The model under review builds one solid part; all positions refer to its coordinate system, in mm. A direction names the side the tool comes from. Coordinates: 2 decimals unless noted, no trailing zeros. Loops run counter-clockwise (first coordinate to the right, second up) from the corner with the lowest first, then second, coordinate; pieces in that order, holes last. Notation, with made-up numbers: M -29.75,-36.75 L 9.25,-36.75 A12 ccw 9.25,-23.75 Z; hole C 14.25,25.25 d7. An arc over 180 degrees is marked long. Use one line per item in the form item = value.
```python
from build123d import *

# Parameters (mm, degrees)
F0_W      = 33
F0_H      = 10
F1_DEPTH  = 5
F2_R      = 1.75
F3_DEPTH  = 5
F2_R_2    = 3
F4_DEPTH  = 3
F5_W      = 33
F5_H      = 30
F6_DEPTH  = 6
F7_R      = 4
F8_DEPTH  = 6
F9_R      = 1.5
F10_DEPTH = 4.2929008565
F12_DEPTH = 6


with BuildPart() as f1:
    # F0 (on Front) → F1 (new body)
    with BuildSketch(Plane.XZ):
        Rectangle(F0_W, F0_H)
    extrude(amount=F1_DEPTH)

    # F2 (on face) → F3 (cut, through all)
    with BuildSketch(Plane.XZ.offset(5)):
        with Locations((-12, 1)):
            Circle(F2_R)
        with Locations((12, 1)):
            Circle(F2_R)
    extrude(amount=-F3_DEPTH, mode=Mode.SUBTRACT)

    # F2 (on face) → F4 (cut)
    with BuildSketch(Plane.XZ.offset(5)):
        with Locations((-12, 1)):
            Circle(F2_R_2)
        with Locations((-12, 1)):
            Circle(F2_R, mode=Mode.SUBTRACT)
        with Locations((12, 1)):
            Circle(F2_R_2)
        with Locations((12, 1)):
            Circle(F2_R, mode=Mode.SUBTRACT)
    extrude(amount=-F4_DEPTH, mode=Mode.SUBTRACT)

    # F5 (on face) → F6 (join)
    with BuildSketch(Plane(origin=(0, 0, -5), x_dir=(1, 0, 0), z_dir=(0, 0, -1))):
        with Locations((0, 15)):
            Rectangle(F5_W, F5_H)
    extrude(amount=F6_DEPTH)

    # F7 (on face) → F8 (cut, through all)
    with BuildSketch(Plane.XY.offset(-5)):
        with Locations((0, -22)):
            Circle(F7_R)
    extrude(amount=-F8_DEPTH, mode=Mode.SUBTRACT)

    # F9 (on face) → F10 (cut, through all)
    with BuildSketch(Plane.XZ.offset(30)):
        with Locations((0, -8)):
            Circle(F9_R)
    extrude(amount=-F10_DEPTH, mode=Mode.SUBTRACT)

    # F11 (on face) → F12 (cut, through all)
    with BuildSketch(Plane.XY.offset(-5)):
        with BuildLine():
            Line((12.5, -7), (-12.5, -7))
            Line((-12.5, -7), (-12.5, -14.6550831307))
            Line((-12.5, -14.6550831307), (-12.5, -22))
            Line((-12.5, -22), (-7.5, -22))
            ThreePointArc((-7.5, -22), (0, -14.5), (7.5, -22))
            Line((7.5, -22), (12.5, -22))
            Line((12.5, -22), (12.5, -14.6550831307))
            Line((12.5, -14.6550831307), (12.5, -7))
        make_face()
    extrude(amount=-F12_DEPTH, mode=Mode.SUBTRACT)


solid = f1.part
```
1. The part is to be moulded in two halves that separate along Z. For faces 6 (the face through (0, -15, -11)), 7 (the face through (10, -22, -8)), 8 (the face through (9.6, -3.5, -0.8)), say which applies: pulls with the +Z half, pulls with the -Z half, needs draft (parallel to the pull), parting line crosses it, or undercut.
Response values:
face_6 = pulls with the -Z half
face_7 = needs draft
face_8 = undercut
2. Add section D-D (x = -12). State the section outline as (y, z) points.
Response values:
outline = M -30,-11 L -22,-11 L -22,-5 L -30,-5 Z; M -7,-11 L 0,-11 L 0,-0.75 L -2,-0.75 L -2,-2 L -5,-2 L -5,-5 L -7,-5 Z; M -5,4 L -2,4 L -2,2.75 L 0,2.75 L 0,5 L -5,5 Z
3. Add section C-C (y = -12.5). State the section outline as (x, z) points.
Response values:
outline = M -16.5,-11 L -12.5,-11 L -12.5,-5 L -16.5,-5 Z; M 12.5,-11 L 16.5,-11 L 16.5,-5 L 12.5,-5 Z
4. Wall thickness on line 1 along Z through (x, y) = (12, -3); line 2 along Z through (x, y) = (-12, -1); line 3 along Y through (x, z) = (-11.5, -7.75): over which ranges is each line inside the solid? List them lowest first. Write a range as from..to.
Response values:
line_1 = -11..-2, 4..5
line_2 = -11..-0.75, 2.75..5
line_3 = -30..-22, -7..0
5. Add section A-A (x = 6). State the section outline as (y, z) points.
Response values:
outline = M -30,-11 L -17.5,-11 L -17.5,-5 L -30,-5 Z; M -7,-11 L 0,-11 L 0,5 L -5,5 L -5,-5 L -7,-5 Z
6. Insertion check: P1, Ø1.8, axis at x = 0, z = -8, coming from the -Y side; P2, Ø5, axis at x = -13, z = -0.5, coming from the -Y side; P3, Ø5, axis at x = 0.5, z = -7, coming from the -Y side; P4, Ø1, axis at x = 3.5, y = -25.5, coming from the +Z side. Each pin has a flat end and moves straight along its axis. Give the tip position at first contact, or say it passes through.
Response values:
P1 = -18.1
P2 = -5
P3 = -30
P4 = -5
7. Machinability: for faces 1 (the face through (-10.331, -1.014, 1.526)), 2 (the face through (1.386, -27.884, -8.575)), 3 (the face through (0, -7, -8)), 4 (the face through (0, -5, 0)), 5 (the face through (16.5, -11, -6)), which of the approach directions +Z, -Z, +X, -X, +Y, -Y give a long, thin tool a straight path to every point of the face, cutting with its end or side? Answer none if there is none.
Response values:
face_1 = +Y, -Y
face_2 = -Y
face_3 = +Z, -Z
face_4 = +Z, +X, -X, -Y
face_5 = +Z, -Z, +X, +Y, -Y
8. Add section B-B (z = 1). State the section outline as (x, y) points.
Response values:
outline = M -16.5,-5 L -15,-5 L -15,-2 L -13.75,-2 L -13.75,0 L -16.5,0 Z; M -10.25,-2 L -9,-2 L -9,-5 L 9,-5 L 9,-2 L 10.25,-2 L 10.25,0 L -10.25,0 Z; M 13.75,-2 L 15,-2 L 15,-5 L 16.5,-5 L 16.5,0 L 13.75,0 Z
